```python
from build123d import *

# Parameters (mm, degrees)
F0_R     = 21.720665
F0_R_2   = 16.520494
F1_DEPTH = 38.1
F0_W     = 84.640459
F0_H     = 65.472521
F2_DEPTH = 25.4


with BuildPart() as f1:
    # F0 (on Front) → F1 (new body)
    with BuildSketch(Plane.XZ):
        Circle(F0_R)
        Circle(F0_R_2, mode=Mode.SUBTRACT)
    extrude(amount=F1_DEPTH)

    # F0 (on Front) → F2 (join)
    with BuildSketch(Plane.XZ):
        with Locations((1.507592, -0.216593)):
            Rectangle(F0_W, F0_H)
        Circle(F0_R, mode=Mode.SUBTRACT)
    extrude(amount=F2_DEPTH)


solid = f1.part
```
Work out the finished part from the listing and answer in its coordinate system (mm). A direction names the side the tool comes from. Give positions to 0.01 mm unless a question says otherwise; leave off trailing zeros. Order: outer loops, then holes, each group sorted by start corner. A loop starts at its lowest first (then second) coordinate and runs counter-clockwise, first axis right, second up. Notation, with made-up numbers: (71.5, 57.5) - (101.5, 57.5) arc R8 cw to (101.5, 70.5) - close; hole circle Ø7 at (-28, 47). An arc over 180 degrees is marked (long way). One line per item, written item: value. Start each with the question number.
1. Section B-B, the plane z = 0 is taken. Write down the section's boundary in (x, y), then the cut area to 3 significant figures.
2. Section A-A, the plane x = 0 is taken. Write down the section's boundary in (y, z), then the cut area to 3 significant figures.
3. Section D-D, the plane z = 19.5 is taken. Write down the section's boundary in (x, y).
4. This flat-tipped pin is pushed along its axis until it touches: pin 1 Ø2 at (x, z) = (21.5, -25) entering from -Y. Where does it stop, or does it pass through?
5. Which of the six approach directions +Z, -Z, +X, -X, +Y, -Y give full straight-line access (tool end or side, diameter ignored) to faces 4 (the face through (5, -38.1, 16)), 5 (the face through (1, -25.4, 22))?
6. Section C-C, the plane y = -5.5 is taken. Write down the section's boundary in (x, z), then the cut area to 3 significant figures.
7. Consider line 1 (Z direction, x = 0, y = -10); line 2 (Z direction, x = 0, y = -27); line 3 (Y direction, x = 28, z = -7). Determine where each line is inside the solid, lowest interval first.
8. For a pull along Z with two mould halves and no side action, classify faces 1 (the face through (1, -13, 32.52)), 2 (the face through (43.828, -13, -1)), 3 (the face through (-3.581, -18.783, -16.128)) as released by +Z, released by -Z, zero draft, split by the parting line, or undercut.
Filled sheet:
1. outline: (-40.81, -25.4) - (-21.72, -25.4) - (-21.72, -38.1) - (-16.52, -38.1) - (-16.52, 0) - (-40.81, 0) - close; (16.52, -38.1) - (21.72, -38.1) - (21.72, -25.4) - (43.83, -25.4) - (43.83, 0) - (16.52, 0) - close
1. area: 1,440 mm²
2. outline: (-38.1, -21.72) - (-25.4, -21.72) - (-25.4, -32.95) - (0, -32.95) - (0, -16.52) - (-38.1, -16.52) - close; (-38.1, 16.52) - (0, 16.52) - (0, 32.52) - (-25.4, 32.52) - (-25.4, 21.72) - (-38.1, 21.72) - close
2. area: 956 mm²
3. outline: (-40.81, -25.4) - (-9.57, -25.4) - (-9.57, -38.1) - (9.57, -38.1) - (9.57, -25.4) - (43.83, -25.4) - (43.83, 0) - (-40.81, 0) - close
4. pin 1: y = -25.4
5. face 4: +Z, -Z, +X, -X, -Y
5. face 5: -Y
6. outline: (-40.81, -32.95) - (43.83, -32.95) - (43.83, 32.52) - (-40.81, 32.52) - close; hole circle Ø33.04 at (0, 0)
6. area: 4,680 mm²
7. line 1: -32.95 to -16.52, 16.52 to 32.52
7. line 2: -21.72 to -16.52, 16.52 to 21.72
7. line 3: -25.4 to 0
8. face 1: released by +Z
8. face 2: zero draft
8. face 3: undercut
